Study the drawing (mm; zero at the part's minimum x, y, z) and answer. A direction names the side the tool comes from. Give positions to 0.01 mm unless a question says otherwise; leave off trailing zeros. Order: outer loops, then holes, each group sorted by start corner. A loop starts at its lowest first (then second) coordinate and runs counter-clockwise, first axis right, second up.
Item 1: A cutting plane is placed at C-C (z = 5.5). Write down the section's boundary in (x, y).
Item 2: Given pin 1 Ø6 at (x, z) = (13.5, 4.5) entering from +Y; pin 2 Ø3 at (y, z) = (25, 10.5) entering from +X; pin 3 Ø7.5 at (x, y) = (4.5, 8) entering from +Z; pin 4 Ø4 at (y, z) = (5, 8.5) entering from -X, each flat-ended and moving along its own axis, determine where each tip first touches the part or whether it passes through.
Item 3: Which of the six approach directions +Z, -Z, +X, -X, +Y, -Y give full straight-line access (tool end or side, diameter ignored) to the marked faces 1, 2 and 3?
Item 4: Find the intervals of material crossed by line 1 along Y through (x, z) = (15, 3.1); line 2 along Z through (x, y) = (23.5, 21.75); line 3 along Y through (x, z) = (13.75, 0.75) (1 decimal), in increasing order.
Item 5: A cutting plane is placed at B-B (z = 10). Write down the section's boundary in (x, y), plus the area to 3 significant figures.
Item 6: The mould has two halves that part along Y. Classify the marked faces 4, 5 and 6: +Y half, -Y half, draft (parallel to the pull), parting line (faces both ways), or undercut.
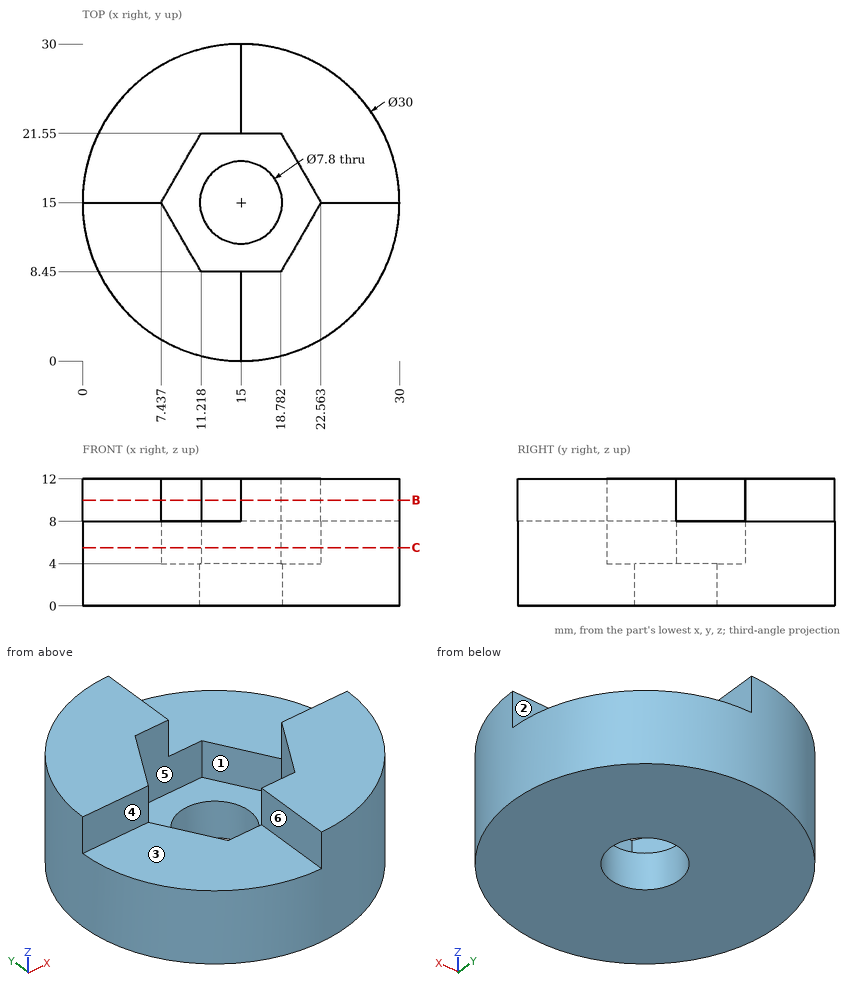
Response values:
1. outline: circle Ø30 at (15, 15); hole (7.44, 15) - (11.22, 8.45) - (18.78, 8.45) - (22.56, 15) - (18.78, 21.55) - (11.22, 21.55) - close
2. pin 1: stops at y = 30
2. pin 2: stops at x = 15
2. pin 3: stops at z = 8
2. pin 4: stops at x = 2.35
3. face 1: +Z
3. face 2: +Z, +X, +Y
3. face 3: +Z, -X, -Y
4. line 1: y = 0 to 11.1, 18.9 to 30
4. line 2: z = 0 to 8
4. line 3: y = 0.1 to 11.3, 18.7 to 29.9
5. outline: (0, 15) - (7.44, 15) - (11.22, 21.55) - (15, 21.55) - (15, 30) arc R15 ccw to start; (15, 0) arc R15 ccw to (30, 15) - (22.56, 15) - (18.78, 8.45) - (15, 8.45) - close
5. area: 279 mm2
6. face 4: -Y half
6. face 5: undercut
6. face 6: draft
